Build history of the part. All positions in model axes, mm. Face numbers are marked on the shaded views. A direction names the side the tool comes from. Give positions to 0.01 mm unless a question says otherwise; leave off trailing zeros. Loops run counter-clockwise (first coordinate to the right, second up) from the corner with the lowest first, then second, coordinate; pieces in that order, holes last. Notation, with made-up numbers: M 1,-34.75 L 12,-34.75 A24 ccw 12,-17.75 Z; hole C 59,75.25 d2. An arc over 180 degrees is marked long. Answer in a Markdown table with one row per item. Add a question column.
```python
from build123d import *

# Parameters (mm, degrees)
F0_W     = 40.0558
F0_H     = 40.0558
F1_DEPTH = 1.7526
F3_R     = 1.7526
F4_DEPTH = 31.75
F5_W     = 40.0558
F5_H     = 40.0558
F6_DEPTH = 0.019685
F7_W     = 40.0558
F7_H     = 44.069
F8_DEPTH = 0.019685


with BuildPart() as f1:
    # F0 (on Top) → F1 (new body, symmetric)
    with BuildSketch(Plane.XY):
        Rectangle(F0_W, F0_H)
    extrude(amount=F1_DEPTH, both=True)

    # F3 (on face) → F4 (join)
    with BuildSketch(Plane(origin=(0, -20.0279, 0), x_dir=(-1, 0, 0), z_dir=(0, 1, 0))):
        with Locations((-18.2753, 0)):
            Circle(F3_R)
        with Locations((18.2753, 0)):
            Circle(F3_R)
    extrude(amount=-F4_DEPTH)


with BuildPart() as f6:
    # F5 (on face) → F6 (new body)
    with BuildSketch(Plane.XY):
        Rectangle(F5_W, F5_H)
    extrude(amount=F6_DEPTH)


with BuildPart() as f8:
    # F7 (on face) → F8 (new body)
    with BuildSketch(Plane(origin=(0, 0, -1.7526), x_dir=(1, 0, 0), z_dir=(0, 0, -1))):
        with Locations((0, 2.0066)):
            Rectangle(F7_W, F7_H)
    extrude(amount=F8_DEPTH)


solid = f1.part
```
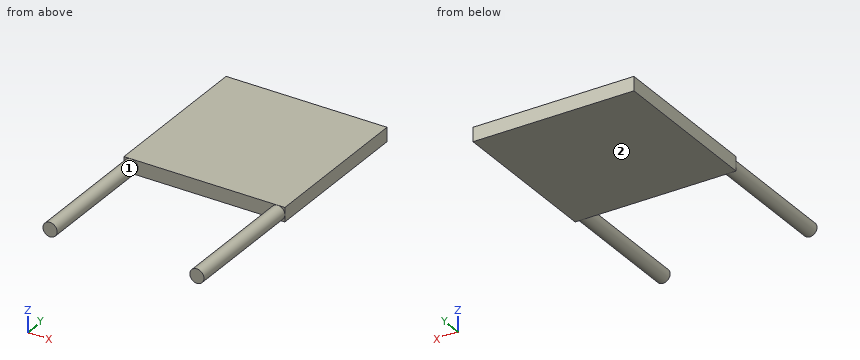
(1) Wall check: line 1 (X direction, y = -28, z = -0.2); line 2 (Y direction, x = -6.5, z = -1.3); line 3 (X direction, y = -26, z = 0.8). Give the ranges that are in metal, low to high.
(2) Tool access for the marked faces 1 and 2: list every direction of +Z, -Z, +X, -X, +Y, -Y with a clear straight run to the whole face (end or side of a thin tool).
(3) Slice it at B-B, the plane x = 13. Give the cut face in (y, z), then the cut area to 3 significant figures.
(4) Pin check, flat tip, straight feed: pin 1 (1.8 mm diameter, centred on x = 3.5, z = 1, fed in from -Y). Stop position of the tip, or through.
(5) Slice it at A-A, the plane z = -1.05. Give the cut face in (x, y).
(6) Slice it at C-C, the plane y = -30. Give the cut face in (x, z).
Solution:
| question | item | result |
|---|---|---|
| 1 | line 1 | -20.02 to -16.53, 16.53 to 20.02 |
| 1 | line 2 | -20.03 to 20.03 |
| 1 | line 3 | -19.83 to -16.72, 16.72 to 19.83 |
| 2 | face 1 | -Y |
| 2 | face 2 | -Z, +X, -X, +Y, -Y |
| 3 | outline | M -20.03,-1.75 L 20.03,-1.75 L 20.03,1.75 L -20.03,1.75 Z |
| 3 | area | 140 mm^2 |
| 4 | pin 1 | y = -20.03 |
| 5 | outline | M -20.03,-20.03 L -19.68,-20.03 L -19.68,-51.78 L -16.87,-51.78 L -16.87,-20.03 L 16.87,-20.03 L 16.87,-51.78 L 19.68,-51.78 L 19.68,-20.03 L 20.03,-20.03 L 20.03,20.03 L -20.03,20.03 Z |
| 6 | outline | C -18.28,0 d3.51; C 18.28,0 d3.51 |
